Design review of the part built by this model. Coordinates are the model's own, in mm. A direction names the side the tool comes from. Round coordinates to 2 decimals unless told otherwise and drop trailing zeros. Loops run counter-clockwise (first coordinate to the right, second up) from the corner with the lowest first, then second, coordinate; pieces in that order, holes last. Notation, with made-up numbers: (40, 56) - (83, 56) arc R18 cw to (83, 86) - close; hole circle Ø4 at (37, 50.5). An arc over 180 degrees is marked (long way). Return JSON: item names as keys, results as strings. Group by question number.
(1) Wall thickness on L1, parallel to X at y = 4.5, z = -12; L2, parallel to Z at x = -7.5, y = 3; L3, parallel to X at y = 5, z = 14.2: over which ranges is each line inside the solid? List them lowest first. Write a range as [from, to].
(2) For faces 3 (the cylindrical face through (6, 5, 8)), 4 (the flat face through (-13.1, 5, 0)), 5 (the cylindrical face through (0, 7, -8)), 6 (the flat face through (-8, 7.3, 12.25)), list the 3-axis set-ups (+Z, -Z, +X, -X, +Y, -Y) from which the entire face can be reached by the end or side of a thin tool; tool diameter is ignored.
(3) We need section D-D, the plane x = -5.5. Write out the cut boundary in (y, z).
(4) The part is to be moulded in two halves that separate along Y. For faces 1 (the flat face through (0, 7.3, 12.25)), 2 (the flat face through (8, 5, 7)), say which applies: pulls with the +Y half, pulls with the -Y half, needs draft (parallel to the pull), parting line crosses it, or undercut.
(5) We need section B-B, the plane z = 10. Write out the cut boundary in (x, y).
(6) We need section A-A, the plane x = 0. Give the number of separate pieces and of enclosed holes in the cut face, and give its area (3 significant figures).
(7) Clearance check with a flat-ended pin moving along its axis: pin 1 (3 mm diameter, centred on x = -8, y = 5, fed in from +Z). State where the tip first meets the part, or that it passes through.
Autodesk Inventor part; units mm, degrees
ref_plane "YZ Plane" through (0, 0, 0) normal (1, 0, 0) x (0, 1, 0)
ref_plane "XZ Plane" through (0, 0, 0) normal (0, 1, 0) x (-1, 0, 0)
ref_plane "XY Plane" through (0, 0, 0) normal (0, 0, 1) x (1, 0, 0)
sketch "Эскиз1" plane through (0, 0, 0) normal (0, 1, 0) x (-1, 0, 0)
  line L0 (-13.1, 17) -> (13.1, 17)
  line L1 (13.1, 17) -> (13.1, -17)
  line L2 (13.1, -17) -> (-13.1, -17)
  line L3 (-13.1, -17) -> (-13.1, 17)
  line L4 (-13.1, 17) -> (13.1, -17) construction
  line L5 (13.1, 17) -> (-13.1, -17) construction
  point P0 (0, 0)
  dimension "d0" = 26.2
  dimension "d1" = 34
extrude "Выдавливание1" add sketch "Эскиз1" along normal blind 10
sketch "Эскиз2" plane through (-13.1, 0, 17) normal (0, 0, 1) x (1, 0, 0)
  line L0 (0, 10) -> (26.2, 10)
  line L1 (13.1, 10) -> (13.1, 5)
  circle A0 centre (13.1, 5) radius 2
  point P0 (13.1, 0)
  dimension "d4" = 5
  dimension "d5" = 4
extrude "Выдавливание2" cut sketch "Эскиз2" against normal blind 10
sketch "Эскиз4" plane through (0, 10, 0) normal (0, 1, 0) x (1, 0, 0)
  line L0 (2, -7) -> (-2, -7)
  line L1 (3.4971, -12.25) -> (-3.4971, -12.25)
  line L2 (-3.4971, -12.25) -> (-3.4971, -8.75)
  line L3 (-3.4971, -8.75) -> (3.4971, -8.75)
  line L4 (3.4971, -8.75) -> (3.4971, -12.25)
  line L5 (3.4971, -12.25) -> (-3.4971, -8.75) construction
  line L6 (-3.4971, -12.25) -> (3.4971, -8.75) construction
  point P0 (0, 0)
  point P1 (0, -10.5)
  dimension "d20" = 10.5
extrude "Выдавливание3" cut sketch "Эскиз4" against normal through all
pattern_linear "Прямоуг.массив2" count 3 spacing 8 along (1, 0, 0) of "Выдавливание2", "Выдавливание3" first direction both ways yes
mirror "Зеркальное отражение2" about plane through (0, 0, 0) normal (0, 0, 1) of "Выдавливание2", "Выдавливание3", "Прямоуг.массив2"
sketch "Эскиз5" plane through (0, 10, 0) normal (0, 1, 0) x (1, 0, 0)
  circle A0 centre (0, 0) radius 5
  dimension "d17" = 10
extrude "Выдавливание4" cut sketch "Эскиз5" against normal blind 10
sketch "Эскиз6" plane through (0, 10, 0) normal (0, 1, 0) x (1, 0, 0)
  circle A0 centre (0, 0) radius 5
  line L0 (4.5029, 8.75) -> (4.5029, 12.25)
  line L1 (4.5029, 12.25) -> (11.4971, 12.25)
  line L2 (11.4971, 12.25) -> (11.4971, 8.75)
  line L3 (-11.4971, 8.75) -> (-11.4971, 12.25)
  line L4 (-11.4971, 12.25) -> (-4.5029, 12.25)
  line L5 (-4.5029, 12.25) -> (-4.5029, 8.75)
  line L6 (-3.4971, 8.75) -> (-3.4971, 12.25)
  line L7 (-3.4971, 12.25) -> (3.4971, 12.25)
  line L8 (3.4971, 12.25) -> (3.4971, 8.75)
  line L9 (4.5029, -12.25) -> (4.5029, -8.75)
  line L10 (11.4971, -8.75) -> (11.4971, -12.25)
  line L11 (11.4971, -12.25) -> (4.5029, -12.25)
  line L12 (-11.4971, -12.25) -> (-11.4971, -8.75)
  line L13 (-4.5029, -8.75) -> (-4.5029, -12.25)
  line L14 (-4.5029, -12.25) -> (-11.4971, -12.25)
  line L15 (3.4971, -8.75) -> (3.4971, -12.25)
  line L16 (3.4971, -12.25) -> (-3.4971, -12.25)
  line L17 (-3.4971, -12.25) -> (-3.4971, -8.75)
  line L18 (-13.1, -17) -> (13.1, -17)
  line L19 (13.1, -17) -> (13.1, 17)
  line L20 (13.1, 17) -> (-13.1, 17)
  line L21 (-13.1, 17) -> (-13.1, -17)
  line L22 (11.4971, 8.75) -> (4.5029, 8.75)
  line L23 (-4.5029, 8.75) -> (-11.4971, 8.75)
  line L24 (3.4971, 8.75) -> (-3.4971, 8.75)
  line L25 (4.5029, -8.75) -> (11.4971, -8.75)
  line L26 (-11.4971, -8.75) -> (-4.5029, -8.75)
  line L27 (-3.4971, -8.75) -> (3.4971, -8.75)
properties part number "000.406 - Проставка" material "Пластик АБС"
Solutions:
{
 "1": {"L1": "[-13.1, -11.5], [-4.5, -3.5], [3.5, 4.5], [11.5, 13.1]", "L2": "[-17, -12.25], [-8.75, 8.75], [12.25, 17]", "L3": "[-13.1, -10], [-6, -2], [2, 6], [10, 13.1]"},
 "2": {"face 3": "+Z", "face 4": "+Z, -Z, -X, +Y, -Y", "face 5": "-Z", "face 6": "+Y, -Y"},
 "3": {"outline": "(0, -17) - (10, -17) - (10, -12.25) - (0, -12.25) - close; (0, -8.75) - (10, -8.75) - (10, 8.75) - (0, 8.75) - close; (0, 12.25) - (10, 12.25) - (10, 17) - (0, 17) - close"},
 "4": {"face 1": "needs draft", "face 2": "undercut"},
 "5": {"outline": "(-13.1, 0) - (-11.5, 0) - (-11.5, 10) - (-13.1, 10) - close; (-4.5, 0) - (-3.5, 0) - (-3.5, 10) - (-4.5, 10) - close; (3.5, 0) - (4.5, 0) - (4.5, 10) - (3.5, 10) - close; (11.5, 0) - (13.1, 0) - (13.1, 10) - (11.5, 10) - close"},
 "6": {"separate pieces": "6", "enclosed holes": "0", "area": "118 mm^2"},
 "7": {"pin 1": "z = 7"}
}
